Read the model definition and answer for the solid it produces. Units are mm, in the model's axes. A direction names the side the tool comes from. Coordinates: 2 decimals unless noted, no trailing zeros. Loops run counter-clockwise (first coordinate to the right, second up) from the corner with the lowest first, then second, coordinate; pieces in that order, holes last. Notation, with made-up numbers: (-39.75, 42) -> (0.25, 42) arc R22 cw to (0.25, 66) -> close; hole circle Ø4 at (-4.5, 71.5). An arc over 180 degrees is marked (long way). One line per question, with ' | ' between items. Start each with the question number.
```python
from build123d import *

# Parameters (mm, degrees)
SKETCH_1_R      = 2.5
EXTRUDE_1_DEPTH = 100
EXTRUDE_2_DEPTH = 3
SKETCH_3_R      = 1.5
EXTRUDE_3_DEPTH = 10
EXTRUDE_4_DEPTH = 3


with BuildPart() as part:
    # 草圖1 → 填料-伸長1 (new body)
    with BuildSketch(Plane(origin=(0, 0, 0), x_dir=(0, 0, -1), z_dir=(1, 0, 0))):
        Circle(SKETCH_1_R)
    extrude(amount=EXTRUDE_1_DEPTH)

    # 草圖2 → 填料-伸長2 (add)
    with BuildSketch(Plane(origin=(100, 0, 0), x_dir=(0, 0, -1), z_dir=(1, 0, 0))):
        with BuildLine():
            Line((-1.930937659, 1.587916798), (0.609729217, 4.677417052))
            ThreePointArc((0.609729217, 4.677417052), (4.128583674, 5.020437914), (4.471604535, 1.501583457))
            Line((4.471604535, 1.501583457), (1.930937659, -1.587916798))
            ThreePointArc((1.930937659, -1.587916798), (-1.587916798, -1.930937659), (-1.930937659, 1.587916798))
        make_face()
    extrude(amount=EXTRUDE_2_DEPTH)

    # 草圖3 → 填料-伸長3 (add)
    with BuildSketch(Plane(origin=(103, 0, 0), x_dir=(0, 0, -1), z_dir=(1, 0, 0))):
        with Locations((2.540666876, 3.089500255)):
            Circle(SKETCH_3_R)
    extrude(amount=EXTRUDE_3_DEPTH)

    # 草圖4 → 填料-伸長4 (add)
    with BuildSketch(Plane(origin=(0, 0, 0), x_dir=(0, 0, -1), z_dir=(1, 0, 0))):
        Polygon((-3.149027259, -2.533172054), (0.619277721, -3.993723631), (3.76830498, -1.460551577), (3.149027259, 2.533172054), (-0.619277721, 3.993723631), (-3.76830498, 1.460551577), align=None)
    extrude(amount=-EXTRUDE_4_DEPTH)


solid = part.part
```
(1) Find the intervals of material crossed by probe 1 along X at (y, z) = (3, -0.5); probe 2 along Y at (x, z) = (44.5, 0); probe 3 along X at (y, z) = (-0.25, 1.75), in increasing order. Write a range as from..to.
(2) A tool of negligible diameter and unlimited length cuts with its end or side. For faces 1 (the flat face through (-1.479, 3.253, -1.291)), 2 (the flat face through (101.48, 3.11, 0.68)), 3 (the flat face through (101.48, -0.02, -3.22)), 4 (the flat face through (103, 2, -1)), from which of +Z, -Z, +X, -X, +Y, -Y can it reach the whole face along a straight path? Write none if from no direction.
(3) Each of these flat-tipped pins is pushed along its axis until it touches: pin 1 Ø5 at (x, z) = (93.5, -3) entering from +Y; pin 2 Ø1.5 at (x, y) = (30.5, 0) entering from +Z; pin 3 Ø5 at (x, z) = (12.5, -2.5) entering from +Y. Where does it stop, or does it pass through?
(4) Section A-A on y = 0 is taken. Write down the section's boundary in (x, z).
(5) Section B-B on x = 57 is taken. Write down the section's boundary in (y, z).
Working result:
1) probe 1: x = -3..0, 100..103 | probe 2: y = -2.5..2.5 | probe 3: x = -3..103
2) face 1: -Z, -X, +Y | face 2: +Z, +X, +Y | face 3: -Z, +X, -Y | face 4: +X
3) pin 1: stops at y = 2.45 | pin 2: stops at z = 2.5 | pin 3: stops at y = 2.5
4) outline: (-3, -3.54) -> (0, -3.54) -> (0, -2.5) -> (100, -2.5) -> (100, -3.24) -> (103, -3.24) -> (103, 2.5) -> (0, 2.5) -> (0, 3.54) -> (-3, 3.54) -> close
5) outline: circle Ø5 at (0, 0)
